Here's how the part is built. I have some questions about the finished solid (model axes, mm). Round coordinates to 2 decimals unless told otherwise and drop trailing zeros. Loops run counter-clockwise (first coordinate to the right, second up) from the corner with the lowest first, then second, coordinate; pieces in that order, holes last. Notation, with made-up numbers: M -32.75,76.5 L 24.25,76.5 A25 ccw 24.25,112.5 Z; hole C -40,-7.75 d3. An arc over 180 degrees is marked long. One line per question, with ' | ' between items. Start each with the question number.
```python
from build123d import *

# Parameters (mm, degrees)
BOSS_EXTRUDE1_DEPTH = 2.5


# Read off the part's stored shape, not the designer's step: M4 Clearance Hole1
with BuildPart() as part:
    # Sketch1 → Boss-Extrude1 (new body)
    with BuildSketch(Plane(origin=(0, 0, 0), x_dir=(1, 0, 0), z_dir=(0, 1, 0))):
        with BuildLine():
            Line((-25, 5), (25, 5))
            ThreePointArc((25, 5), (30, 0), (25, -5))
            Line((25, -5), (-25, -5))
            ThreePointArc((-25, -5), (-30, 0), (-25, 5))
        make_face()
    extrude(amount=BOSS_EXTRUDE1_DEPTH)

    # M4 Clearance Hole1 outline → M4 Clearance Hole1 (revolve, cut)
    with BuildSketch(Plane(origin=(-25, 0, 0), x_dir=(1, 0, 0), z_dir=(0, 0, 1))):
        Polygon((0, 0), (2.25, 0), (2.25, 2.479022509), (2.275, 2.5), (0, 2.5), align=None)
    revolve(axis=Axis((-25, 0, 0), (0, 1, 0)), mode=Mode.SUBTRACT)

    # M4 Clearance Hole1 2 outline → M4 Clearance Hole1 2 (revolve, cut)
    with BuildSketch(Plane(origin=(25, 0, 0), x_dir=(1, 0, 0), z_dir=(0, 0, 1))):
        Polygon((0, 0), (2.25, 0), (2.25, 2.479022509), (2.275, 2.5), (0, 2.5), align=None)
    revolve(axis=Axis((25, 0, 0), (0, 1, 0)), mode=Mode.SUBTRACT)


solid = part.part
```
1) Please list where these lines run through material, in increasing order: L1, parallel to X at y = 1.5, z = 0; L2, parallel to Z at x = -25, y = 1.5; L3, parallel to X at y = 1.6, z = 1.5. Write a range as from..to.
2) Imagine slicing it at A-A (z = 0). Write out the boundary of the cut face in (x, y) (3 decimals), then the cut area to 3 significant figures.
3) I'm going to push a flat-ended pin straight in: pin 1 Ø4 at (x, z) = (21, 4) entering from -Y. Where does the tip first touch, or does it pass through?
4) We'd pull the mould along X, two halves only. Please class faces 1 (the face through (-22.854, 1.257, -0.676)), 2 (the face through (0, 1, 5)), 3 (the face through (30, 1, 0)): pulls with the +X half, pulls with the -X half, needs draft (parallel to the pull), parting line crosses it, or undercut.
5) Imagine slicing it at B-B (y = 1.05). Write out the boundary of the cut face in (x, z).
Results are:
1) L1: -30..-27.25, -22.75..22.75, 27.25..30 | L2: -5..-2.25, 2.25..5 | L3: -29.77..-26.68, -23.32..23.32, 26.68..29.77
2) outline: M -30,0 L -27.25,0 L -27.25,2.479 L -27.275,2.5 L -30,2.5 Z; M -22.75,0 L 22.75,0 L 22.75,2.479 L 22.725,2.5 L -22.725,2.5 L -22.75,2.479 Z; M 27.25,0 L 30,0 L 30,2.5 L 27.275,2.5 L 27.25,2.479 Z | area: 127 mm²
3) pin 1: y = 0
4) face 1: undercut | face 2: needs draft | face 3: pulls with the +X half
5) outline: M -25,-5 L 25,-5 A5 ccw 25,5 L -25,5 A5 ccw Z; hole C -25,0 d4.5; hole C 25,0 d4.5
